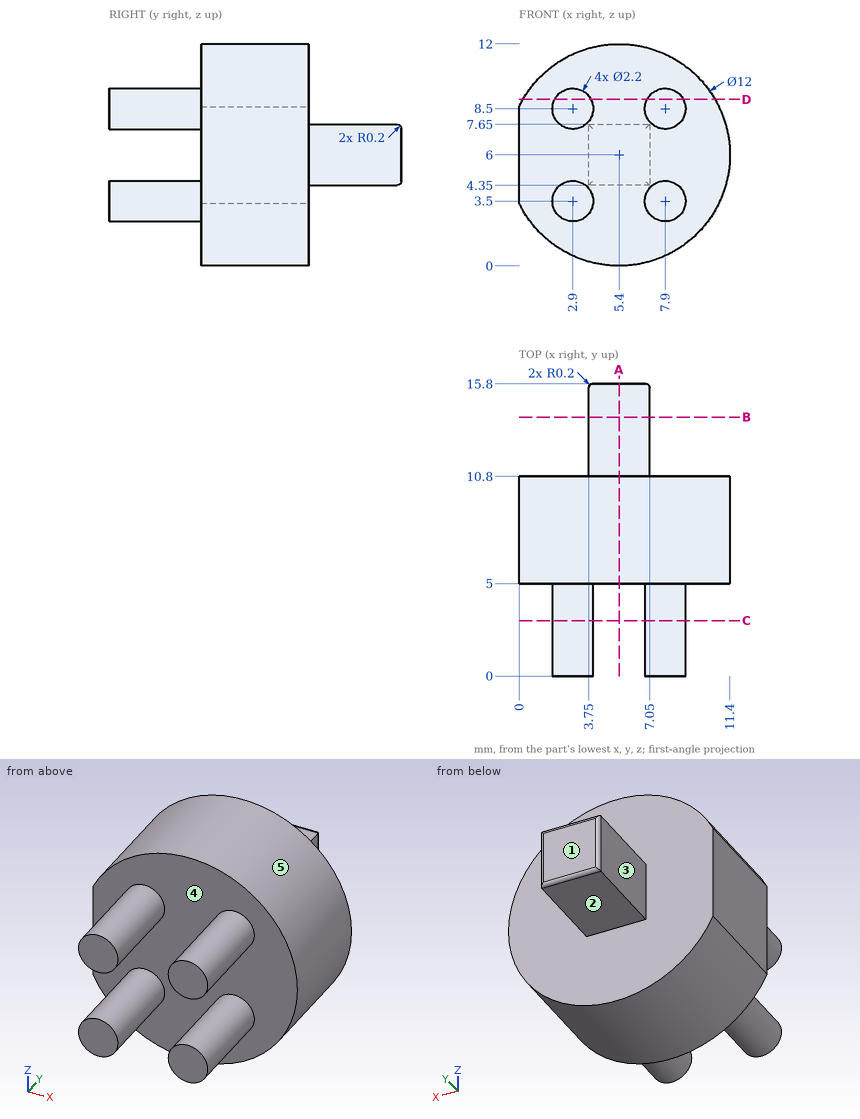
For this review, use the dimensioned drawing (mm, ordinates from the lowest corner) and the shaded views. A direction names the side the tool comes from. Round coordinates to 2 decimals unless told otherwise and drop trailing zeros. Order: outer loops, then holes, each group sorted by start corner. A loop starts at its lowest first (then second) coordinate and runs counter-clockwise, first axis right, second up.
1) Machinability: for the marked faces 1, 2, 3, 4 and 5, which of the approach directions +Z, -Z, +X, -X, +Y, -Y give a long, thin tool a straight path to every point of the face, cutting with its end or side? Answer none if there is none.
The answers:
face 1: +Z, -Z, +X, -X, +Y
face 2: -Z, +X, -X, +Y
face 3: +Z, -Z, -X, +Y
face 4: -Y
face 5: +Y, -Y
2) Clearance check with flat-ended pins moving along their axes: pin 1 Ø1.5 at (x, y) = (7.5, 3) entering from +Z; pin 2 Ø3 at (x, z) = (9, 10) entering from -Y; pin 3 Ø1 at (x, y) = (6.5, 12) entering from -Z; pin 4 Ø1.6 at (x, y) = (5, 13.5) entering from +Z. State where each tip first meets the part, or that it passes through.
The answers:
pin 1: stops at z = 9.6
pin 2: stops at y = 0
pin 3: stops at z = 4.35
pin 4: stops at z = 7.65
3) Consider section B-B (y = 14). State the section outline as (x, z) points.
The answers:
outline: (3.75, 4.35) - (7.05, 4.35) - (7.05, 7.65) - (3.75, 7.65) - close
4) Consider section D-D (z = 9). State the section outline as (x, y) points.
The answers:
outline: (0.2, 5) - (1.92, 5) - (1.92, 0) - (3.88, 0) - (3.88, 5) - (6.92, 5) - (6.92, 0) - (8.88, 0) - (8.88, 5) - (10.6, 5) - (10.6, 10.8) - (0.2, 10.8) - close
5) For L1, parallel to X at y = 3.5, z = 3.5; L2, parallel to Y at x = 1, z = 2.5; L3, parallel to Z at x = 6.25, y = 12, list the stretches that pass through material, from the lowest coordinate up.
The answers:
L1: x = 1.8 to 4, 6.8 to 9
L2: y = 5 to 10.8
L3: z = 4.35 to 7.65
6) Consider section C-C (y = 3). State the section outline as (x, z) points.
The answers:
outline: circle Ø2.2 at (2.9, 3.5); circle Ø2.2 at (2.9, 8.5); circle Ø2.2 at (7.9, 3.5); circle Ø2.2 at (7.9, 8.5)
7) Consider section A-A (x = 5.4). State the section outline as (y, z) points.
The answers:
outline: (5, 0) - (10.8, 0) - (10.8, 4.35) - (15.6, 4.35) arc R0.2 ccw to (15.8, 4.55) - (15.8, 7.45) arc R0.2 ccw to (15.6, 7.65) - (10.8, 7.65) - (10.8, 12) - (5, 12) - close
